```python
from build123d import *

# Parameters (mm, degrees)
BOSS_EXTRUDE1_DEPTH = 35.56


with BuildPart() as part:
    # Sketch1 → Boss-Extrude1 (new, symmetric)
    with BuildSketch(Plane(origin=(0, 0, 0), x_dir=(1, 0, 0), z_dir=(0, 1, 0))):
        Polygon((7.69896584, 0), (3.84948292, 6.6675), (-3.84948292, 6.6675), (-7.69896584, 0), (-3.84948292, -6.6675), (3.84948292, -6.6675), align=None)
    extrude(amount=BOSS_EXTRUDE1_DEPTH, both=True)

    # Loft2: read off the stored shape, not the designer's step
    # Loft2: loft between two sections, ruled curve by curve
    loft2_from = [
        Edge.make_bspline([(25.4, 45.75948292, 6.6675), (25.4, 47.042643893, 6.6675), (25.4, 48.325804866, 6.6675), (25.4, 50.892126813, 6.6675), (25.4, 52.175287786, 6.6675), (25.4, 53.458448759, 6.6675)], [0, 0, 0, 0, 0.5, 0.5, 1, 1, 1, 1], 3),
        Edge.make_bspline([(25.4, 53.458448759, 6.6675), (25.4, 54.100029246, 5.55625), (25.4, 54.741609733, 4.445), (25.4, 56.024770706, 2.2225), (25.4, 56.666351193, 1.11125), (25.4, 57.307931679, 0)], [0, 0, 0, 0, 0.5, 0.5, 1, 1, 1, 1], 3),
        Edge.make_bspline([(25.4, 41.91, 0), (25.4, 42.551580487, 1.11125), (25.4, 43.193160973, 2.2225), (25.4, 44.476321947, 4.445), (25.4, 45.117902433, 5.55625), (25.4, 45.75948292, 6.6675)], [0, 0, 0, 0, 0.5, 0.5, 1, 1, 1, 1], 3),
        Edge.make_bspline([(25.4, 57.307931679, 0), (25.4, 56.666351193, -1.11125), (25.4, 56.024770706, -2.2225), (25.4, 54.741609733, -4.445), (25.4, 54.100029246, -5.55625), (25.4, 53.458448759, -6.6675)], [0, 0, 0, 0, 0.5, 0.5, 1, 1, 1, 1], 3),
        Edge.make_bspline([(25.4, 53.458448759, -6.6675), (25.4, 52.175287786, -6.6675), (25.4, 50.892126813, -6.6675), (25.4, 48.325804866, -6.6675), (25.4, 47.042643893, -6.6675), (25.4, 45.75948292, -6.6675)], [0, 0, 0, 0, 0.5, 0.5, 1, 1, 1, 1], 3),
        Edge.make_bspline([(25.4, 45.75948292, -6.6675), (25.4, 45.117902433, -5.55625), (25.4, 44.476321947, -4.445), (25.4, 43.193160973, -2.2225), (25.4, 42.551580487, -1.11125), (25.4, 41.91, 0)], [0, 0, 0, 0, 0.5, 0.5, 1, 1, 1, 1], 3),
    ]
    loft2_to = [
        Edge.make_bspline([(-7.69896584, 35.56, 0), (-7.057385353, 35.56, -1.11125), (-6.415804866, 35.56, -2.2225), (-5.132643893, 35.56, -4.445), (-4.491063406, 35.56, -5.55625), (-3.84948292, 35.56, -6.6675)], [0, 0, 0, 0, 0.5, 0.5, 1, 1, 1, 1], 3),
        Edge.make_bspline([(-3.84948292, 35.56, -6.6675), (-2.566321947, 35.56, -6.6675), (-1.283160973, 35.56, -6.6675), (1.283160973, 35.56, -6.6675), (2.566321947, 35.56, -6.6675), (3.84948292, 35.56, -6.6675)], [0, 0, 0, 0, 0.5, 0.5, 1, 1, 1, 1], 3),
        Edge.make_bspline([(-3.84948292, 35.56, 6.6675), (-4.491063406, 35.56, 5.55625), (-5.132643893, 35.56, 4.445), (-6.415804866, 35.56, 2.2225), (-7.057385353, 35.56, 1.11125), (-7.69896584, 35.56, 0)], [0, 0, 0, 0, 0.5, 0.5, 1, 1, 1, 1], 3),
        Edge.make_bspline([(3.84948292, 35.56, -6.6675), (4.491063406, 35.56, -5.55625), (5.132643893, 35.56, -4.445), (6.415804866, 35.56, -2.2225), (7.057385353, 35.56, -1.11125), (7.69896584, 35.56, 0)], [0, 0, 0, 0, 0.5, 0.5, 1, 1, 1, 1], 3),
        Edge.make_bspline([(7.69896584, 35.56, 0), (7.057385353, 35.56, 1.11125), (6.415804866, 35.56, 2.2225), (5.132643893, 35.56, 4.445), (4.491063406, 35.56, 5.55625), (3.84948292, 35.56, 6.6675)], [0, 0, 0, 0, 0.5, 0.5, 1, 1, 1, 1], 3),
        Edge.make_bspline([(3.84948292, 35.56, 6.6675), (2.566321947, 35.56, 6.6675), (1.283160973, 35.56, 6.6675), (-1.283160973, 35.56, 6.6675), (-2.566321947, 35.56, 6.6675), (-3.84948292, 35.56, 6.6675)], [0, 0, 0, 0, 0.5, 0.5, 1, 1, 1, 1], 3),
    ]
    loft2 = Solid(Shell([*[Face.make_surface_from_curves(loft2_from[k], loft2_to[k]) for k in range(6)], Face(Wire(loft2_from)), Face(Wire(loft2_to))]))
    add(loft2)


solid = part.part
```
Geometry check sheet. Reference: the model listing, model coordinates, mm. A direction names the side the tool comes from. Give positions to 0.01 mm unless a question says otherwise; leave off trailing zeros. Write each loop counter-clockwise with the first axis right and the second up, starting at its lowest first coordinate (ties: lowest second). Pieces come first, ordered by that corner, then holes.
1) Section check A-A, the plane y = -10.5. Record the boundary of the cut face in (x, z), and give its area (3 significant figures).
2) Access from +Z, -Z, +X, -X, +Y, -Y to the whole of each face (thin tool, end or side, straight path). Record for faces 1 (the flat face through (5.8, 0.5, -3.29)), 2 (the flat face through (0, 0, 6.668)), 3 (the flat face through (5.747, 0.498, 3.38)).
3) Material ranges on L1, parallel to Z at x = -6, y = 21; L2, parallel to Y at x = 7.5, z = -4.5; L3, parallel to Y at x = 6, z = -3.5, recorded low to high.
4) Gauge pin test, flat ends, axial feed: pin 1 (2 mm diameter, centred on y = -21.5, z = 1.5, fed in from -X); pin 2 (5 mm diameter, centred on x = 18.5, z = -0.5, fed in from +Y); pin 3 (3 mm diameter, centred on x = 19, z = 3.5, fed in from +Y). Record the tip position at first contact, or that the pin passes through.
Computed:
1. outline: (-7.7, 0) - (-3.85, -6.67) - (3.85, -6.67) - (7.7, 0) - (3.85, 6.67) - (-3.85, 6.67) - close
1. area: 154 mm2
2. face 1: -Z, +X, -Y
2. face 2: +Z, +X, -X, +Y, -Y
2. face 3: +Z, +X, -Y
3. L1: z = -2.94 to 2.94
3. L2: y = 38.22 to 40.71
3. L3: y = 35.89 to 40.89
4. pin 1: stops at x = -7.41
4. pin 2: stops at y = 52.72
4. pin 3: stops at y = 50.94
